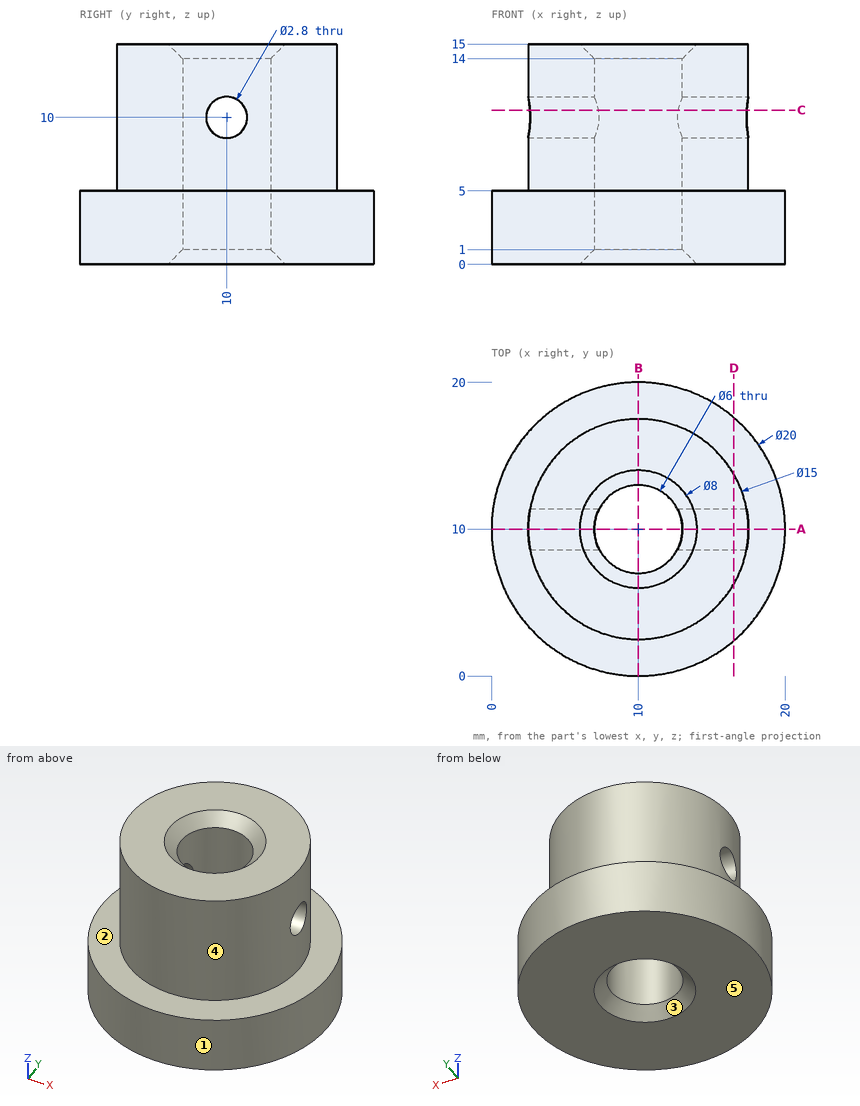
For this review, use the dimensioned drawing (mm, ordinates from the lowest corner) and the shaded views. A direction names the side the tool comes from. Round coordinates to 2 decimals unless told otherwise and drop trailing zeros. Write each loop counter-clockwise with the first axis right and the second up, starting at its lowest first coordinate (ties: lowest second). Pieces come first, ordered by that corner, then holes. Notation, with made-up numbers: (60.5, -4.5) - (89.5, -4.5) arc R9 ccw to (89.5, 7.5) - close; hole circle Ø5 at (10.25, 22). An arc over 180 degrees is marked (long way). Answer as a JSON object with one key per item and string values.
1. To check wall thickness, follow line 1 along Z through (x, y) = (14.9, 10); line 2 along Y through (x, z) = (10, 5.5); line 3 along Z through (x, y) = (18.25, 14). State the ranges of each line that lie inside material, in increasing order.
Response values:
{"line 1": "z = 0 to 8.6, 11.4 to 15", "line 2": "y = 2.5 to 7, 13 to 17.5", "line 3": "z = 0 to 5"}
2. We need section D-D on x = 16.5. Give the boundary of the cut face in (y, z).
Response values:
{"outline": "(2.4, 0) - (17.6, 0) - (17.6, 5) - (13.74, 5) - (13.74, 15) - (6.26, 15) - (6.26, 5) - (2.4, 5) - close; hole circle Ø2.8 at (10, 10)"}
3. We need section B-B on x = 10. Give the boundary of the cut face in (y, z), then the cut area to 3 significant figures.
Response values:
{"outline": "(0, 0) - (6, 0) - (7, 1) - (7, 14) - (6, 15) - (2.5, 15) - (2.5, 5) - (0, 5) - close; (13, 1) - (14, 0) - (20, 0) - (20, 5) - (17.5, 5) - (17.5, 15) - (14, 15) - (13, 14) - close", "area": "158 mm2"}
4. We need section C-C on z = 10.5. Give the boundary of the cut face in (x, y).
Response values:
{"outline": "(2.61, 8.69) arc R7.5 ccw to (17.39, 8.69) - (12.7, 8.69) arc R3 cw to (7.3, 8.69) - close; (2.61, 11.31) - (7.3, 11.31) arc R3 cw to (12.7, 11.31) - (17.39, 11.31) arc R7.5 ccw to start"}
5. Draft analysis for pull direction Y (two halves, no side actions). For the marked faces 3, 4 and 5, state which applies: +Y half, -Y half, draft (parallel to the pull), parting line (faces both ways), or undercut.
Response values:
{"face 3": "undercut", "face 4": "parting line", "face 5": "draft"}
6. Tool access review of the marked faces 1 and 2: name each direction out of +Z, -Z, +X, -X, +Y, -Y from which nothing blocks a thin tool from reaching the whole face with its end or side.
Response values:
{"face 1": "+Z, -Z", "face 2": "+Z"}
7. We need section A-A on y = 10. Give the boundary of the cut face in (x, z), then the cut area to 3 significant figures.
Response values:
{"outline": "(0, 0) - (6, 0) - (7, 1) - (7, 8.6) - (2.5, 8.6) - (2.5, 5) - (0, 5) - close; (2.5, 11.4) - (7, 11.4) - (7, 14) - (6, 15) - (2.5, 15) - close; (13, 1) - (14, 0) - (20, 0) - (20, 5) - (17.5, 5) - (17.5, 8.6) - (13, 8.6) - close; (13, 11.4) - (17.5, 11.4) - (17.5, 15) - (14, 15) - (13, 14) - close", "area": "133 mm2"}
8. For pin 1 Ø8 at (x, z) = (11.5, 13) entering from -Y; pin 2 Ø5 at (x, z) = (3, 10) entering from +Y; pin 3 Ø4 at (x, z) = (7, 10) entering from -Y; pin 4 Ø6 at (y, z) = (10.5, 1.5) entering from -X, all flat-tipped, find the tip position at first contact; note any pin that passes through.
Response values:
{"pin 1": "stops at y = 2.5", "pin 2": "stops at y = 16", "pin 3": "stops at y = 2.57", "pin 4": "stops at x = 0"}
